Can you work these out from the model? Positions are in its coordinate system, mm. A direction names the side the tool comes from. Round coordinates to 2 decimals unless told otherwise and drop trailing zeros. Loops run counter-clockwise (first coordinate to the right, second up) from the corner with the lowest first, then second, coordinate; pieces in that order, holes last. Notation, with made-up numbers: (-27, -6.75) - (22, -6.75) arc R27 ccw to (22, 13.25) - close; hole circle Ø7 at (89, 28). An arc over 180 degrees is marked (long way). Answer as CSV lines item,"result".
```python
from build123d import *

# Parameters (mm, degrees)
F0_R           = 203.2
F1_DEPTH       = 4.7625
F2_R           = 203.2
F3_DEPTH       = 4.7625
F4_R           = 152.4
F5_DEPTH       = 19.05
F6_W           = 4.7625
F6_H           = 158.7546515355
F7_DEPTH       = 19.05
F10_DEPTH      = 19.05
F10_DEPTH_BACK = 19.05


with BuildPart() as f1:
    # F0 (on Front) → F1 (new body)
    with BuildSketch(Plane.XZ):
        Circle(F0_R)
        with BuildLine():
            ThreePointArc((-86.9334783468, -125.1732013753), (-131.9822715367, -76.2), (-151.8699114374, -12.7))
            Line((-151.8699114374, -12.7), (-21.9970452561, -12.7))
            Line((-21.9970452561, -12.7), (-86.9334783468, -125.1732013753))
        make_face(mode=Mode.SUBTRACT)
        with BuildLine():
            ThreePointArc((64.9364330906, -137.8732013753), (0, -152.4), (-64.9364330906, -137.8732013753))
            Line((-64.9364330906, -137.8732013753), (0, -25.4))
            Line((0, -25.4), (64.9364330906, -137.8732013753))
        make_face(mode=Mode.SUBTRACT)
        with BuildLine():
            Line((21.9970452561, -12.7), (151.8699114374, -12.7))
            ThreePointArc((151.8699114374, -12.7), (131.9822715367, -76.2), (86.9334783468, -125.1732013753))
            Line((86.9334783468, -125.1732013753), (21.9970452561, -12.7))
        make_face(mode=Mode.SUBTRACT)
        with BuildLine():
            ThreePointArc((-151.8699114374, 12.7), (-131.9822715367, 76.2), (-86.9334783468, 125.1732013753))
            Line((-86.9334783468, 125.1732013753), (-21.9970452561, 12.7))
            Line((-21.9970452561, 12.7), (-151.8699114374, 12.7))
        make_face(mode=Mode.SUBTRACT)
        with BuildLine():
            ThreePointArc((-64.9364330906, 137.8732013753), (0, 152.4), (64.9364330906, 137.8732013753))
            Line((64.9364330906, 137.8732013753), (0, 25.4))
            Line((0, 25.4), (-64.9364330906, 137.8732013753))
        make_face(mode=Mode.SUBTRACT)
        with BuildLine():
            ThreePointArc((86.9334783468, 125.1732013753), (131.9822715367, 76.2), (151.8699114374, 12.7))
            Line((151.8699114374, 12.7), (21.9970452561, 12.7))
            Line((21.9970452561, 12.7), (86.9334783468, 125.1732013753))
        make_face(mode=Mode.SUBTRACT)
    extrude(amount=F1_DEPTH)

    # F2 (on face) → F3 (join)
    with BuildSketch(Plane(origin=(0, 0, 0), x_dir=(-1, 0, 0), z_dir=(0, 1, 0))):
        Circle(F2_R)
    extrude(amount=F3_DEPTH)

    # F4 (on face) → F5 (join)
    with BuildSketch(Plane(origin=(0, 4.7625, 0), x_dir=(-1, 0, 0), z_dir=(0, 1, 0))):
        Circle(F4_R)
    extrude(amount=F5_DEPTH)

    # F6 (on face) → F7 (cut, through all)
    with BuildSketch(Plane(origin=(0, 23.8125, 0), x_dir=(-1, 0, 0), z_dir=(0, 1, 0))):
        with Locations((0, 123.8087211165)):
            Rectangle(F6_W, F6_H)
        Polygon((-37.2880920976, 24.2779206671), (-174.7736532963, 103.6552464349), (-177.1549032963, 99.5308004494), (-39.6693420976, 20.1534746816), align=None)
        Polygon((-39.6693420976, -20.1534746816), (-177.1549032963, -99.5308004494), (-174.7736532963, -103.6552464349), (-37.2880920976, -24.2779206671), align=None)
        with Locations((0, -123.8087211165)):
            Rectangle(F6_W, F6_H)
        Polygon((37.2880920976, -24.2779206671), (174.7736532963, -103.6552464349), (177.1549032963, -99.5308004494), (39.6693420976, -20.1534746816), align=None)
        Polygon((39.6693420976, 20.1534746816), (177.1549032963, 99.5308004494), (174.7736532963, 103.6552464349), (37.2880920976, 24.2779206671), align=None)
    extrude(amount=-F7_DEPTH, mode=Mode.SUBTRACT)

    # F9: F1 across plane


with BuildPart() as f1_1:
    add(f1.part)
    add(f1.part.mirror(Plane(origin=(0, 23.8125, 0), x_dir=(-1, 0, 0), z_dir=(0, 1, 0))))

    # F6 (on face) → F10 (join, two sides)
    with BuildSketch(Plane(origin=(0, 23.8125, 0), x_dir=(-1, 0, 0), z_dir=(0, 1, 0))) as f10_sk:
        with Locations((0, 123.8087211165)):
            Rectangle(F6_W, F6_H)
        Polygon((-37.2880920976, 24.2779206671), (-174.7736532963, 103.6552464349), (-177.1549032963, 99.5308004494), (-39.6693420976, 20.1534746816), align=None)
        Polygon((-39.6693420976, -20.1534746816), (-177.1549032963, -99.5308004494), (-174.7736532963, -103.6552464349), (-37.2880920976, -24.2779206671), align=None)
        with Locations((0, -123.8087211165)):
            Rectangle(F6_W, F6_H)
        Polygon((37.2880920976, -24.2779206671), (174.7736532963, -103.6552464349), (177.1549032963, -99.5308004494), (39.6693420976, -20.1534746816), align=None)
        Polygon((39.6693420976, 20.1534746816), (177.1549032963, 99.5308004494), (174.7736532963, 103.6552464349), (37.2880920976, 24.2779206671), align=None)
    extrude(amount=-F10_DEPTH)
    extrude(f10_sk.sketch, amount=F10_DEPTH_BACK)


solid = f1_1.part
```
Q1. On a 3-axis mill with a long thin cutter (end or side, diameter ignored), from which of +Z, -Z, +X, -X, +Y, -Y can I reach the whole of each face in a straight line? I mean faces 3 (the flat face through (88, 47.625, 57)), 4 (the flat face through (1, 0, 104)), 5 (the flat face through (169, 4.762, 1)). Say none if no direction works.
Checks:
face 3,"+Y"
face 4,"-Y"
face 5,"+X"
Q2. If I drill on line 1 along Z through (x, y) = (-114.5, 49.5); line 2 along Y through (x, z) = (131, -138.5); line 3 along X through (y, z) = (-2, -15.5), over which ranges is the centre line in solid material (lowest first)? Write a range as [from, to].
Checks:
line 1,"[-167.87, -100.58], [-12.7, 12.7], [100.58, 167.87]"
line 2,"[-4.76, 4.76], [42.86, 52.39]"
line 3,"[-202.61, -151.61], [-23.61, 23.61], [151.61, 202.61]"
Q3. We'd pull the mould along X, two halves only. Please class faces 1 (the flat face through (-175, 42.862, 1)), 2 (the cylindrical face through (131.51, 49.97, 77.01)): pulls with the +X half, pulls with the -X half, needs draft (parallel to the pull), parting line crosses it, or undercut.
Checks:
face 1,"needs draft"
face 2,"undercut"
Q4. Imagine slicing it at A-A (z = -158). Write out the boundary of the cut face in (x, y).
Checks:
outline,"(-127.77, -4.76) - (127.77, -4.76) - (127.77, 4.76) - (2.38, 4.76) - (2.38, 42.86) - (127.77, 42.86) - (127.77, 52.39) - (-127.77, 52.39) - (-127.77, 42.86) - (-2.38, 42.86) - (-2.38, 4.76) - (-127.77, 4.76) - close"
Q5. Imagine slicing it at B-B (z = 143). Write out the boundary of the cut face in (x, y) (1 decimal).
Checks:
outline,"(-144.4, -4.8) - (-52.7, -4.8) - (-52.7, 0) - (52.7, 0) - (52.7, -4.8) - (144.4, -4.8) - (144.4, 4.8) - (52.7, 4.8) - (52.7, 42.9) - (144.4, 42.9) - (144.4, 52.4) - (52.7, 52.4) - (52.7, 47.6) - (-52.7, 47.6) - (-52.7, 52.4) - (-144.4, 52.4) - (-144.4, 42.9) - (-52.7, 42.9) - (-52.7, 4.8) - (-144.4, 4.8) - close"
Q6. I'm going to push flat-ended pins straight in: pin 1 Ø1 at (x, z) = (49.5, 15) entering from -Y; pin 2 Ø5 at (x, y) = (-71, -1.5) entering from -Z; pin 3 Ø3 at (x, y) = (87.5, 13.5) entering from -Z; pin 4 Ø2.5 at (x, z) = (176.5, 101.5) entering from -Y. Where does each tip first touch, or does it pass through?
Checks:
pin 1,"y = 0"
pin 2,"z = -191.31"
pin 3,"z = -125.82"
pin 4,"y = -4.76"
